Check sheet for the modelled part. Datum: model origin and axes. Units: mm. Face numbers are marked on the shaded views. A direction names the side the tool comes from. Round coordinates to 2 decimals unless told otherwise and drop trailing zeros. Write each loop counter-clockwise with the first axis right and the second up, starting at its lowest first coordinate (ties: lowest second). Pieces come first, ordered by that corner, then holes.
Item 1: Set-up check for the marked faces 1 and 2: record each of +Z, -Z, +X, -X, +Y, -Y from which the full face is reachable in a straight line by a thin tool's end or side.
Item 2: Section check A-A, the plane x = -28.5. Record the cut outline in (y, z), plus the area to 3 significant figures.
Item 3: Section check B-B, the plane y = 4.5. Record the cut outline in (x, z), plus the area to 3 significant figures.
Item 4: Material ranges on line 1 along Y through (x, z) = (-107, -18); line 2 along Z through (x, y) = (35, 15.75); line 3 along Y through (x, z) = (-80, 0.55), recorded low to high.
Item 5: Depth check by flat-ended pin: pin 1 (4 mm diameter, centred on x = 74, z = -14, fed in from +Y); pin 2 (3.5 mm diameter, centred on x = -100, z = -13.75, fed in from -Y); pin 3 (7.5 mm diameter, centred on x = 19.5, y = 12, fed in from -Z). Enter the tip coordinate at first touch or a pass-through.
Item 6: Section check C-C, the plane z = -3.5. Record the cut outline in (x, y).
from build123d import *

# Parameters (mm, degrees)
SKETCH1_W                    = 236
SKETCH1_H                    = 26
BASE_FLANGE1_DEPTH           = 1.2
EDGE_FLANGE1_STRIP_W         = 7.8
EDGE_FLANGE1_STRIP_H         = 1.2
EDGE_FLANGE1_STRIP_CUT_DEPTH = 236
EDGE_FLANGE1_DEPTH           = 236
SKETCH9_R                    = 1.5
CUT_EXTRUDE1_DEPTH           = 10
SKETCH10_R                   = 1.5
CUT_EXTRUDE2_DEPTH           = 10


# Sheet-metal steps are written as plain solids
with BuildPart() as part:
    # Sketch1 → Base-Flange1 (new body)
    with BuildSketch(Plane(origin=(0, 0, 0), x_dir=(1, 0, 0), z_dir=(0, 1, 0))):
        with Locations((0, 13)):
            Rectangle(SKETCH1_W, SKETCH1_H)
    extrude(amount=-BASE_FLANGE1_DEPTH)

    # Edge-Flange1 strip (across the edge) → Edge-Flange1 strip cut (cut)
    with BuildSketch(Plane(origin=(-118, 0, 0), x_dir=(0, 0, -1), z_dir=(1, 0, 0))):
        with Locations((-2.4, -0.6)):
            Rectangle(EDGE_FLANGE1_STRIP_W, EDGE_FLANGE1_STRIP_H)
    extrude(amount=EDGE_FLANGE1_STRIP_CUT_DEPTH, mode=Mode.SUBTRACT)

    # Edge-Flange1 section (across the edge) → Edge-Flange1 (add)
    with BuildSketch(Plane(origin=(-118, 0, 0), x_dir=(0, 0, -1), z_dir=(1, 0, 0))):
        with BuildLine():
            Line((-1.2, 1.5), (-1.2, 26))
            Line((-1.2, 26), (0, 26))
            Line((0, 26), (0, 1.5))
            ThreePointArc((0, 1.5), (0.439339828, 0.439339828), (1.5, 0))
            Line((1.5, 0), (1.5, -1.2))
            ThreePointArc((1.5, -1.2), (-0.409188309, -0.409188309), (-1.2, 1.5))
        make_face()
    extrude(amount=EDGE_FLANGE1_DEPTH)

    # Sketch9 → Cut-Extrude1 (cut)
    with BuildSketch(Plane.XZ.offset(1.2)):
        with Locations(Location((-100, -13.75, 0), (0, 0, 270))):
            Circle(SKETCH9_R)
        with Locations(Location((-80, -13.75, 0), (0, 0, 270))):
            Circle(SKETCH9_R)
        with Locations(Location((-60, -13.75, 0), (0, 0, 270))):
            Circle(SKETCH9_R)
        with Locations(Location((-40, -13.75, 0), (0, 0, 270))):
            Circle(SKETCH9_R)
        with Locations(Location((-20, -13.75, 0), (0, 0, 270))):
            Circle(SKETCH9_R)
        with Locations(Location((0, -13.75, 0), (0, 0, 270))):
            Circle(SKETCH9_R)
        with Locations(Location((20, -13.75, 0), (0, 0, 270))):
            Circle(SKETCH9_R)
        with Locations(Location((40, -13.75, 0), (0, 0, 270))):
            Circle(SKETCH9_R)
        with Locations(Location((60, -13.75, 0), (0, 0, 270))):
            Circle(SKETCH9_R)
        with Locations(Location((80, -13.75, 0), (0, 0, 270))):
            Circle(SKETCH9_R)
        with Locations(Location((100, -13.75, 0), (0, 0, 270))):
            Circle(SKETCH9_R)
    extrude(amount=-CUT_EXTRUDE1_DEPTH, mode=Mode.SUBTRACT)

    # Sketch10 → Cut-Extrude2 (cut)
    with BuildSketch(Plane.XY.offset(1.2)):
        with Locations((-100, 13.75)):
            Circle(SKETCH10_R)
        with Locations((-80, 13.75)):
            Circle(SKETCH10_R)
        with Locations((-60, 13.75)):
            Circle(SKETCH10_R)
        with Locations((-40, 13.75)):
            Circle(SKETCH10_R)
        with Locations((-20, 13.75)):
            Circle(SKETCH10_R)
        with Locations((0, 13.75)):
            Circle(SKETCH10_R)
        with Locations((20, 13.75)):
            Circle(SKETCH10_R)
        with Locations((40, 13.75)):
            Circle(SKETCH10_R)
        with Locations((60, 13.75)):
            Circle(SKETCH10_R)
        with Locations((80, 13.75)):
            Circle(SKETCH10_R)
        with Locations((100, 13.75)):
            Circle(SKETCH10_R)
    extrude(amount=-CUT_EXTRUDE2_DEPTH, mode=Mode.SUBTRACT)


solid = part.part
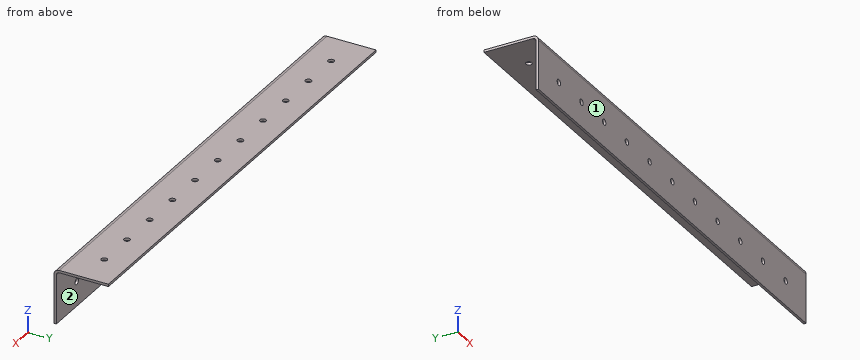
Values found:
1. face 1: +Z, -Z, +X, -X, -Y
1. face 2: -Z, +X, -X, +Y
2. outline: (-1.2, -26) - (0, -26) - (0, -1.5) arc R1.5 cw to (1.5, 0) - (26, 0) - (26, 1.2) - (1.5, 1.2) arc R2.7 ccw to (-1.2, -1.5) - close
2. area: 62.8 mm2
3. outline: (-118, 0) - (118, 0) - (118, 1.2) - (-118, 1.2) - close
3. area: 283 mm2
4. line 1: y = -1.2 to 0
4. line 2: z = 0 to 1.2
4. line 3: y = -0.26 to 12.25, 15.25 to 26
5. pin 1: stops at y = 0
5. pin 2: stops at y = -1.2
5. pin 3: stops at z = 0
6. outline: (-118, -1.2) - (118, -1.2) - (118, 0) - (-118, 0) - close
